Design review of the part built by this model. Coordinates are the model's own, in mm. A direction names the side the tool comes from. Coordinates: 2 decimals unless noted, no trailing zeros. Order: outer loops, then holes, each group sorted by start corner. A loop starts at its lowest first (then second) coordinate and runs counter-clockwise, first axis right, second up. Notation, with made-up numbers: (48, 45) - (94, 45) arc R35 cw to (94, 79) - close; hole circle Ø6 at (63.25, 40.5). An arc over 180 degrees is marked (long way). Write each question's results on one line, items separated by ' | '. Start each with the question number.
```python
from build123d import *

# Parameters (mm, degrees)
BOSS_EXTRUDE1_DEPTH = 20
SKETCH2_R           = 5.65
BOSS_EXTRUDE2_DEPTH = 1.5
SKETCH3_R           = 3.95
BOSS_EXTRUDE3_DEPTH = 7
SKETCH4_R           = 5.65
BOSS_EXTRUDE4_DEPTH = 2.25
SKETCH5_R           = 3.95
BOSS_EXTRUDE5_DEPTH = 7.5
SKETCH9_W           = 25
SKETCH9_H           = 7.5
BOSS_EXTRUDE8_DEPTH = 23
CUT_EXTRUDE1_DEPTH  = 20
CUT_EXTRUDE2_REACH  = 173.135
SKETCH12_W          = 4
SKETCH12_H          = 5
CUT_EXTRUDE3_REACH  = 173.135
SKETCH14_W          = 65
SKETCH14_H          = 10
SKETCH14_W_2        = 117


with BuildPart() as part:
    # Sketch1 → Boss-Extrude1 (new body)
    with BuildSketch(Plane(origin=(0, 0, 0), x_dir=(1, 0, 0), z_dir=(0, 1, 0))):
        Polygon((-6.25, 80), (6.25, 80), (6.25, 0), (6.25, -160), (-6.25, -160), align=None)
    extrude(amount=BOSS_EXTRUDE1_DEPTH)

    # Sketch2 → Boss-Extrude2 (add)
    with BuildSketch(Plane.XY.offset(160)):
        with Locations(Location((0, 10, 0), (0, 0, 180))):
            Circle(SKETCH2_R)
    extrude(amount=BOSS_EXTRUDE2_DEPTH)

    # Sketch3 → Boss-Extrude3 (add)
    with BuildSketch(Plane.XY.offset(161.5)):
        with Locations(Location((0, 10, 0), (0, 0, 180))):
            Circle(SKETCH3_R)
    extrude(amount=BOSS_EXTRUDE3_DEPTH)

    # Sketch4 → Boss-Extrude4 (add)
    with BuildSketch(Plane.ZY.offset(6.25)):
        with Locations(Location((0, 10, 0), (0, 0, 180))):
            Circle(SKETCH4_R)
    boss_extrude4 = extrude(amount=BOSS_EXTRUDE4_DEPTH)

    # Sketch5 → Boss-Extrude5 (add)
    with BuildSketch(Plane.ZY.offset(8.5)):
        with Locations((0, 10)):
            Circle(SKETCH5_R)
    boss_extrude5 = extrude(amount=BOSS_EXTRUDE5_DEPTH)

    # Mirror1: Boss-Extrude4, Boss-Extrude5 across plane
    add(boss_extrude4.mirror(Plane(origin=(0, 0, 0), x_dir=(0, 0, 1), z_dir=(1, 0, 0))))
    add(boss_extrude5.mirror(Plane(origin=(0, 0, 0), x_dir=(0, 0, 1), z_dir=(1, 0, 0))))

    # Sketch9 → Boss-Extrude8 (add)
    with BuildSketch(Plane.XY.offset(160)):
        with Locations((0, -3.75)):
            Rectangle(SKETCH9_W, SKETCH9_H)
    extrude(amount=-BOSS_EXTRUDE8_DEPTH)

    # Sketch10 → Cut-Extrude1 (cut)
    with BuildSketch(Plane.XY.offset(160)):
        Polygon((-10, -5.75), (-10, -3.25), (10, -3.25), (10, -5.75), (7.5, -5.75), (7.5, -7.5), (-7.5, -7.5), (-7.5, -5.75), align=None)
    extrude(amount=-CUT_EXTRUDE1_DEPTH, mode=Mode.SUBTRACT)

    # Sketch12 → Cut-Extrude2 (cut, up to next)
    with BuildSketch(Plane.ZY.offset(6.25), mode=Mode.PRIVATE) as cut_extrude2_sk1:
        with Locations((15, 5)):
            Rectangle(SKETCH12_W, SKETCH12_H)
    cut_extrude2_tool1 = extrude(cut_extrude2_sk1.sketch, amount=-CUT_EXTRUDE2_REACH, mode=Mode.PRIVATE) & part.part
    add(cut_extrude2_tool1.solids().sort_by_distance((-6.25, 5, 15))[0], mode=Mode.SUBTRACT)

    # Sketch14 → Cut-Extrude3 (cut, up to next)
    with BuildSketch(Plane.ZY.offset(6.25), mode=Mode.PRIVATE) as cut_extrude3_sk1:
        with Locations((-47.5, 15)):
            Rectangle(SKETCH14_W, SKETCH14_H)
    cut_extrude3_tool1 = extrude(cut_extrude3_sk1.sketch, amount=-CUT_EXTRUDE3_REACH, mode=Mode.PRIVATE) & part.part
    # Sketch14 → Cut-Extrude3 (cut, up to next)
    with BuildSketch(Plane.ZY.offset(6.25), mode=Mode.PRIVATE) as cut_extrude3_sk2:
        with Locations((78.5, 15)):
            Rectangle(SKETCH14_W_2, SKETCH14_H)
    cut_extrude3_tool2 = extrude(cut_extrude3_sk2.sketch, amount=-CUT_EXTRUDE3_REACH, mode=Mode.PRIVATE) & part.part
    add(cut_extrude3_tool1.solids().sort_by_distance((-6.25, 15, -47.5))[0], mode=Mode.SUBTRACT)
    add(cut_extrude3_tool2.solids().sort_by_distance((-6.25, 15, 78.5))[0], mode=Mode.SUBTRACT)


solid = part.part
```
(1) Mouldability with a two-part tool opening along X and no side actions: class faces 1 (the face through (0, 15, 137)), 2 (the face through (0, -5, 140)), 3 (the face through (-16, 10, 0)) as +X half, -X half, draft (parallel to the pull), parting line (faces both ways), or undercut.
(2) Take a section at D-D (z = 54). State the section outline as (x, y) points, plus the area to 3 significant figures.
(3) Take a section at B-B (z = 145). State the section outline as (x, y) points, plus the area to 3 significant figures.
(4) Tool access review of faces 4 (the face through (0.856, 13.856, 164.951)), 5 (the face through (0, 15, 20)), 6 (the face through (-9, 0, 149)), 7 (the face through (0, 10, -48)), 8 (the face through (12.198, 6.144, -0.856)): name each direction out of +Z, -Z, +X, -X, +Y, -Y from which nothing blocks a thin tool from reaching the whole face with its end or side.
(5) To check wall thickness, follow line 1 along Z through (x, y) = (0, 12.5); line 2 along Z through (x, y) = (3.5, 14.75); line 3 along X through (y, z) = (3, 114). State the ranges of each line that lie inside material, in increasing order. Write a range as [from, to].
(6) Clearance check with flat-ended pins moving along their axes: pin 1 (4 mm diameter, centred on x = 0, z = 101, fed in from +Y); pin 2 (4 mm diameter, centred on x = 5.5, y = -4, fed in from +Z); pin 3 (6 mm diameter, centred on x = 0.5, z = 14, fed in from -Y). State where each tip first meets the part, or that it passes through.
(7) Take a section at A-A (x = 0). State the section outline as (y, z) points, plus the area to 3 significant figures.
(8) Take a section at C-C (z = 0). State the section outline as (x, y) points, plus the area to 3 significant figures.
Worked out:
1) face 1: draft | face 2: undercut | face 3: -X half
2) outline: (-6.25, 0) - (6.25, 0) - (6.25, 10) - (-6.25, 10) - close | area: 125 mm^2
3) outline: (-12.5, -7.5) - (-7.5, -7.5) - (-7.5, -5.75) - (-10, -5.75) - (-10, -3.25) - (10, -3.25) - (10, -5.75) - (7.5, -5.75) - (7.5, -7.5) - (12.5, -7.5) - (12.5, 0) - (6.25, 0) - (6.25, 20) - (-6.25, 20) - (-6.25, 0) - (-12.5, 0) - close | area: 361 mm^2
4) face 4: +Z | face 5: +X, -X, +Y | face 6: +Z, -Z, -X, +Y | face 7: -Z, +X, -X, +Y | face 8: +X
5) line 1: [-15, 20], [137, 168.5] | line 2: [-15, 20], [137, 160] | line 3: [-6.25, 6.25]
6) pin 1: y = 10 | pin 2: z = 160 | pin 3: y = 0
7) outline: (-7.5, 137) - (0, 137) - (0, -80) - (10, -80) - (10, -15) - (20, -15) - (20, 20) - (10, 20) - (10, 137) - (20, 137) - (20, 160) - (15.65, 160) - (15.65, 161.5) - (13.95, 161.5) - (13.95, 168.5) - (6.05, 168.5) - (6.05, 161.5) - (4.35, 161.5) - (4.35, 160) - (-3.25, 160) - (-3.25, 140) - (-7.5, 140) - close; hole (2.5, 13) - (7.5, 13) - (7.5, 17) - (2.5, 17) - close | area: 3,120 mm^2
8) outline: (-16, 6.05) - (-8.5, 6.05) - (-8.5, 4.35) - (-6.25, 4.35) - (-6.25, 0) - (6.25, 0) - (6.25, 4.35) - (8.5, 4.35) - (8.5, 6.05) - (16, 6.05) - (16, 13.95) - (8.5, 13.95) - (8.5, 15.65) - (6.25, 15.65) - (6.25, 20) - (-6.25, 20) - (-6.25, 15.65) - (-8.5, 15.65) - (-8.5, 13.95) - (-16, 13.95) - close | area: 419 mm^2
